```python
from build123d import *

# Parameters (mm, degrees)
SCHIZZO1_R                   = 40
ESTRUSIONE_ESTRUSIONE1_DEPTH = 10
SCHIZZO2_R                   = 25
ESTRUSIONE_ESTRUSIONE2_DEPTH = 40
TAGLIO_ESTRUSIONE1_DEPTH     = 40
NERVATURA16_START            = -5
NERVATURA16_DEPTH            = 10
RIPETIZIONECIRCOLARE1_COUNT  = 4


with BuildPart() as part:
    # Schizzo1 → Estrusione-Estrusione1 (new body)
    with BuildSketch(Plane(origin=(0, 0, 0), x_dir=(1, 0, 0), z_dir=(0, 1, 0))):
        with Locations(Location((0, 0, 0), (0, 0, 270))):
            Circle(SCHIZZO1_R)
    extrude(amount=ESTRUSIONE_ESTRUSIONE1_DEPTH)

    # Schizzo2 → Estrusione-Estrusione2 (add)
    with BuildSketch(Plane(origin=(0, 10, 0), x_dir=(1, 0, 0), z_dir=(0, 1, 0))):
        with Locations(Location((0, 0, 0), (0, 0, 270))):
            Circle(SCHIZZO2_R)
    extrude(amount=ESTRUSIONE_ESTRUSIONE2_DEPTH)

    # Schizzo3 → Taglio-Estrusione1 (cut)
    with BuildSketch(Plane(origin=(0, 50, 0), x_dir=(1, 0, 0), z_dir=(0, 1, 0))):
        with BuildLine():
            Line((-3.349661481, 12.042830563), (-3.349661481, 16.050123743))
            Line((-3.349661481, 16.050123743), (3.349661481, 16.050123743))
            Line((3.349661481, 16.050123743), (3.349661481, 12.042830563))
            ThreePointArc((3.349661481, 12.042830563), (0, -12.5), (-3.349661481, 12.042830563))
        make_face()
    extrude(amount=-TAGLIO_ESTRUSIONE1_DEPTH, mode=Mode.SUBTRACT)

    # Nervatura16: read off the stored shape, not the designer's step
    # Nervatura16 outline → Nervatura16 (add)
    with BuildSketch(Plane(origin=(0, 0, 0), x_dir=(0, 0, -1), z_dir=(1, 0, 0)).offset(NERVATURA16_START)):
        Polygon((-24.494897428, 50), (-25, 50), (-38.573669022, 10), (-24.494897428, 10), align=None)
    nervatura16 = extrude(amount=NERVATURA16_DEPTH)

    # RipetizioneCircolare1: Nervatura16 ×4 about axis
    ripetizionecircolare1_axis = Axis((0, 0, 0), (0, 1, 0))
    for i in range(1, RIPETIZIONECIRCOLARE1_COUNT):
        add(nervatura16.rotate(ripetizionecircolare1_axis, i * 360 / RIPETIZIONECIRCOLARE1_COUNT))


solid = part.part
```
Geometry: final body of the model. Coordinates: model frame, mm. A direction names the side the tool comes from. Round coordinates to 2 decimals unless told otherwise and drop trailing zeros. Write each loop counter-clockwise with the first axis right and the second up, starting at its lowest first coordinate (ties: lowest second). Pieces come first, ordered by that corner, then holes. Notation, with made-up numbers: M -7.5,21 L -2.5,21 A15 cw -2.5,30 Z; hole C 67.25,73.5 d7. An arc over 180 degrees is marked long. Answer in a Markdown table with one row per item. Add a question column.
(1) Ray query, L1, parallel to Y at x = 18.5, z = 22; L2, parallel to X at y = 28.5, z = 0; L3, parallel to Z at x = 0, y = 22. Return the intervals inside material, ascending.
(2) Draft query along X for faces 6 (the face through (3.35, 30, -14)), 7 (the face through (17.533, 29.72, 17.822)), 8 (the face through (-17.533, 29.72, -17.822)). Return one class per face: pulls with the +X half, pulls with the -X half, needs draft (parallel to the pull), parting line crosses it, or undercut.
(3) Cut plane B-B, the plane z = 0. Return the cut outline in (x, y).
(4) Cut plane A-A, the plane x = 0. Return the cut outline in (y, z).
(5) Cut plane D-D, the plane y = 7. Return the cut outline in (x, z), then the cut area to 3 significant figures.
(6) Reachability of faces 1 (the face through (-29, 26, -5)), 2 (the face through (-29, 26, 5)), 3 (the face through (0.5, 30.28, 12.49)), 4 (the face through (29, 26, -5)), 5 (the face through (29, 26, 5)) from +Z, -Z, +X, -X, +Y, -Y: full face, straight path, thin tool, end or side. Return the list, or none.
(7) Contact query for flat-ended pins moving along their axis: pin 1 (1.5 mm diameter, centred on x = -2, y = 6, fed in from +Z); pin 2 (12 mm diameter, centred on x = 18, y = 33.5, fed in from -Z); pin 3 (15.5 mm diameter, centred on y = 35, z = -28.5, fed in from -X); pin 4 (8 mm diameter, centred on x = 28, z = 2, fed in from +Y). Output: stop coordinate, or through.
(8) Cut plane C-C, the plane y = 30. Return the cut outline in (x, z), then the cut area to 3 significant figures.
Established:
| question | item | result |
|---|---|---|
| 1 | L1 | 0 to 10 |
| 1 | L2 | -32.3 to -12.5, 12.5 to 32.3 |
| 1 | L3 | -34.5 to -16.05, 12.5 to 34.5 |
| 2 | face 6 | undercut |
| 2 | face 7 | pulls with the +X half |
| 2 | face 8 | pulls with the -X half |
| 3 | outline | M -40,0 L 40,0 L 40,10 L 38.57,10 L 25,50 L 12.5,50 L 12.5,10 L -12.5,10 L -12.5,50 L -25,50 L -38.57,10 L -40,10 Z |
| 4 | outline | M 0,-40 L 10,-40 L 10,-38.57 L 50,-25 L 50,-16.05 L 10,-16.05 L 10,12.5 L 50,12.5 L 50,25 L 10,38.57 L 10,40 L 0,40 Z |
| 5 | outline | C 0,0 d80 |
| 5 | area | 5,030 mm² |
| 6 | face 1 | -Z, -X, +Y |
| 6 | face 2 | +Z, -X, +Y |
| 6 | face 3 | +Y |
| 6 | face 4 | -Z, +X, +Y |
| 6 | face 5 | +Z, +X, +Y |
| 7 | pin 1 | z = 39.98 |
| 7 | pin 2 | z = -21.93 |
| 7 | pin 3 | x = -13.94 |
| 7 | pin 4 | y = 50 |
| 8 | outline | M -31.79,-5 L -24.49,-5 A25 ccw -5,-24.49 L -5,-31.79 L 5,-31.79 L 5,-24.49 A25 ccw 24.49,-5 L 31.79,-5 L 31.79,5 L 24.49,5 A25 ccw 5,24.49 L 5,31.79 L -5,31.79 L -5,24.49 A25 ccw -24.49,5 L -31.79,5 Z; hole M -3.35,-16.05 L 3.35,-16.05 L 3.35,-12.04 A12.5 ccw long -3.35,-12.04 Z |
| 8 | area | 1,730 mm² |
